Could you check a few things on this drawing? It's one solid part, dimensions in mm from its lowest x, y, z. A direction names the side the tool comes from. Round coordinates to 2 decimals unless told otherwise and drop trailing zeros. Loops run counter-clockwise (first coordinate to the right, second up) from the corner with the lowest first, then second, coordinate; pieces in that order, holes last. Notation, with made-up numbers: (71.25, 7.25) -> (119.25, 7.25) arc R18 cw to (119.25, 27.25) -> close; hole circle Ø10 at (66.5, 53). An arc over 180 degrees is marked (long way). Write each question's results on one line, items separated by ' | '.
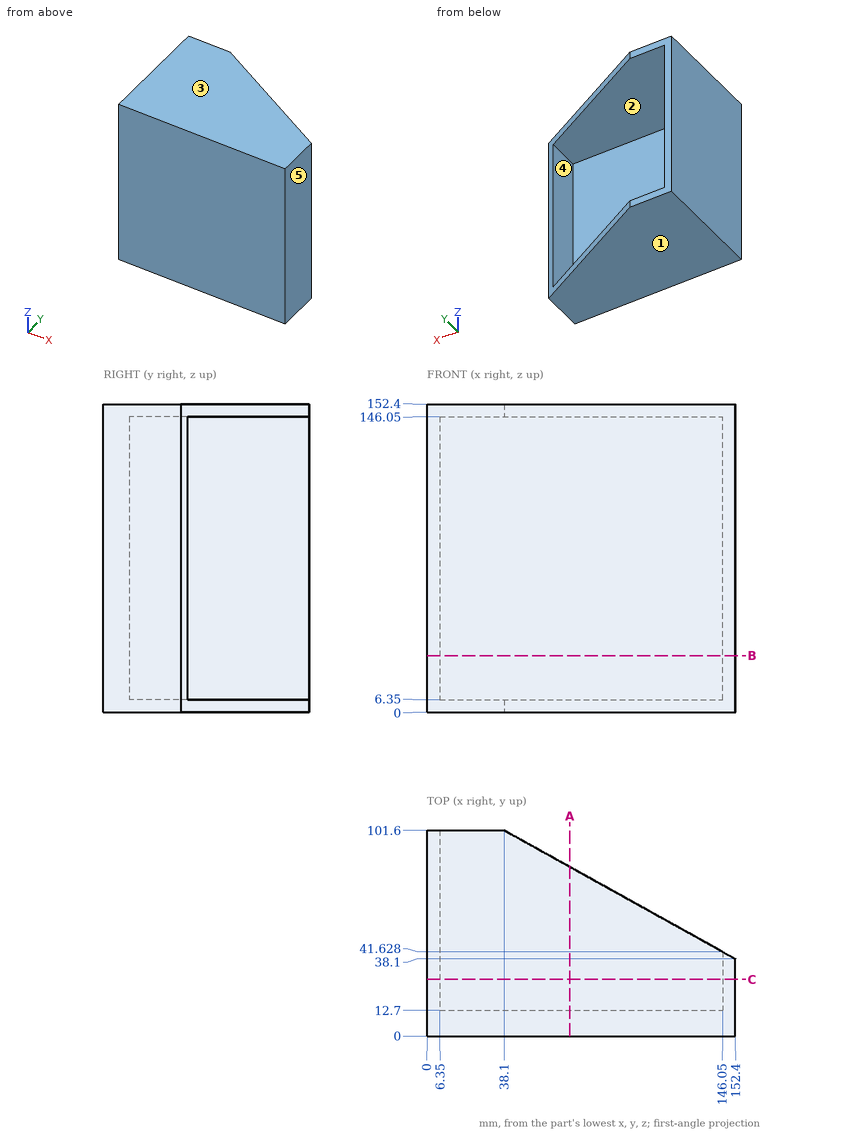
1) If we mould it in two halves opening along X, with no side actions, what happens to the marked faces 3, 4 and 5? For each: released by +X, released by -X, zero draft, split by the parting line, or undercut.
Model answer:
face 3: zero draft | face 4: undercut | face 5: released by +X
2) I want a section at B-B, the plane z = 28. Write out the boundary of the cut face in (x, y), plus the area to 3 significant figures.
Model answer:
outline: (0, 0) -> (152.4, 0) -> (152.4, 38.1) -> (146.05, 41.63) -> (146.05, 12.7) -> (6.35, 12.7) -> (6.35, 101.6) -> (0, 101.6) -> close | area: 2,670 mm2
3) I want a section at C-C, the plane y = 28. Write out the boundary of the cut face in (x, z), plus the area to 3 significant figures.
Model answer:
outline: (0, 0) -> (152.4, 0) -> (152.4, 152.4) -> (0, 152.4) -> close; hole (6.35, 6.35) -> (146.05, 6.35) -> (146.05, 146.05) -> (6.35, 146.05) -> close | area: 3,710 mm2
4) I need wall thicknesses on line 1 (X direction, y = 21, z = 9.5); line 2 (Y direction, x = 79.5, z = 45). Which ranges of each line are inside material? Lowest first, please.
Model answer:
line 1: x = 0 to 6.35, 146.05 to 152.4 | line 2: y = 0 to 12.7
5) For the marked faces 1 and 2, which set-ups out of +Z, -Z, +X, -X, +Y, -Y let a thin tool reach every point of the face, with its end or its side?
Model answer:
face 1: -Z, +X, -X, +Y, -Y | face 2: +Y
6) I'm going to push flat-ended pins straight in: pin 1 (4 mm diameter, centred on y = 83, z = 58, fed in from +X); pin 2 (1.5 mm diameter, centred on x = 134, z = 134, fed in from +Y). Where does each tip first touch, or does it pass through?
Model answer:
pin 1: stops at x = 6.35 | pin 2: stops at y = 12.7
7) I want a section at A-A, the plane x = 70.5. Write out the boundary of the cut face in (y, z).
Model answer:
outline: (0, 0) -> (83.6, 0) -> (83.6, 6.35) -> (12.7, 6.35) -> (12.7, 146.05) -> (83.6, 146.05) -> (83.6, 152.4) -> (0, 152.4) -> close
